```python
from build123d import *

# Parameters (mm, degrees)
F0_R            = 12.7
F1_DEPTH        = 3.175
F3_DEPTH        = 6.35
F3_COPIES_COUNT = 30
F4_R            = 1.5875
F5_DEPTH        = 6.35
F6_R            = 1.5875
F7_DEPTH        = 6.35
F7_COPIES_COUNT = 4


# Not quite as in the source:
# - a pattern or mirror of a feature is missing from the dataset's text; its kind, count and spacing are read off the source's solid
# - a feature names something its author has since deleted; it is built from what else it names


with BuildPart() as f1:
    # F0 (on Front) → F1 (new body, symmetric)
    with BuildSketch(Plane.XZ):
        Circle(F0_R)
    extrude(amount=F1_DEPTH, both=True)

    # F2 (on face) → F3 (join)
    with BuildSketch(Plane.XZ.offset(3.175)):
        Polygon((0, 15.5471283256), (-1.2684115066, 12.6365), (1.2684115066, 12.6365), align=None)
    f3 = extrude(amount=-F3_DEPTH)

    # F3_copies: F3 ×30 about axis
    f3_copies_axis = Axis((0, 0, 0), (0, 1, 0))
    for i in range(1, F3_COPIES_COUNT):
        add(f3.rotate(f3_copies_axis, i * 360 / F3_COPIES_COUNT))

    # F4 (on face) → F5 (cut)
    with BuildSketch(Plane.XZ.offset(3.175)):
        Circle(F4_R)
    extrude(amount=-F5_DEPTH, mode=Mode.SUBTRACT)

    # F6 (on face) → F7 (cut)
    with BuildSketch(Plane.XZ.offset(3.175)):
        with Locations((0, 7.9375)):
            Circle(F6_R)
    f7 = extrude(amount=-F7_DEPTH, mode=Mode.SUBTRACT)

    # F7_copies: F7 ×4 about axis
    f7_copies_axis = Axis((0, 0, 0), (0, 1, 0))
    for i in range(1, F7_COPIES_COUNT):
        add(f7.rotate(f7_copies_axis, i * 360 / F7_COPIES_COUNT), mode=Mode.SUBTRACT)


solid = f1.part
```
Geometry: final body of the model. Coordinates: model frame, mm. A direction names the side the tool comes from. Give positions to 0.01 mm unless a question says otherwise; leave off trailing zeros. Loops run counter-clockwise (first coordinate to the right, second up) from the corner with the lowest first, then second, coordinate; pieces in that order, holes last. Notation, with made-up numbers: (-2.5, 42) -> (21.5, 42) arc R10 cw to (21.5, 52) -> close; hole circle Ø11 at (47.5, -6). An arc over 180 degrees is marked (long way). Return JSON: item names as keys, results as strings.
Item 1: Section A-A, the plane x = -0.5. Output: boundary loops of the cut face in (y, z) (3 decimals), plus the area to 3 significant figures.
Filled in:
{"outline": "(-3.175, -14.4) -> (3.175, -14.4) -> (3.175, -9.444) -> (-3.175, -9.444) -> close; (-3.175, -6.431) -> (3.175, -6.431) -> (3.175, -1.507) -> (-3.175, -1.507) -> close; (-3.175, 1.507) -> (3.175, 1.507) -> (3.175, 6.431) -> (-3.175, 6.431) -> close; (-3.175, 9.444) -> (3.175, 9.444) -> (3.175, 14.4) -> (-3.175, 14.4) -> close", "area": "125 mm^2"}
Item 2: Mould query, pull axis Z, two halves, no side actions, for faces 1 (the flat face through (3, 3.175, 1)), 2 (the flat face through (7.789, -0.044, 11.785)), 3 (the flat face through (-13.228, -0.044, -4.956)). Classes: released by +Z, released by -Z, zero draft, split by the parting line, or undercut.
Filled in:
{"face 1": "zero draft", "face 2": "released by +Z", "face 3": "undercut"}
Item 3: Access query for faces 4 (the flat face through (-12.51, -0.04, -6.48)), 5 (the flat face through (0.643, -0.044, 14.071)), 6 (the flat face through (11.909, -0.044, 7.598)). Directions: +Z, -Z, +X, -X, +Y, -Y. A direction counts if a zero-diameter tool reaches every point of the face in a straight line with its end or side. Return the directions, or none.
Filled in:
{"face 4": "-X, +Y, -Y", "face 5": "+Z, +Y, -Y", "face 6": "+Y, -Y"}
Item 4: Section B-B, the plane y = -2. Count the separate pieces of the cut face and the enclosed holes in it, plus the area to 3 significant figures.
Filled in:
{"separate pieces": "1", "enclosed holes": "5", "area": "575 mm^2"}
Item 5: Pin query (flat end, axial travel): P1, Ø4, axis at x = 0, z = -7.94, coming from the +Y side (3 decimals); P2, Ø2, axis at x = 11, y = 1, coming from the +Z side; P3, Ø3, axis at x = 9.5, y = 1, coming from the -Z side. Return the tip coordinate at first contact, or that it passes through.
Filled in:
{"P1": "y = 3.175", "P2": "z = 10.4", "P3": "z = -12.58"}
Item 6: Line query: line 1 (Z direction, x = 12.5, y = 1.5); line 2 (Z direction, x = -1, y = 1.5); line 3 (X direction, y = -0.75, z = -13.5). Output: solid intervals per line, ascending.
Filled in:
{"line 1": "-7.66 to -6.47, -5.03 to -2.78, -2.56 to 2.56, 2.78 to 5.03, 6.47 to 7.66", "line 2": "-13.25 to -9.17, -6.7 to -1.23, 1.23 to 6.7, 9.17 to 13.25", "line 3": "-6.32 to -5.56, -3.58 to -2.01, -0.89 to 0.89, 2.01 to 3.58, 5.56 to 6.32"}
